```python
from build123d import *

# Parameters (mm, degrees)
SKETCH_1_R               = 32
SKETCH_1_R_2             = 2.5
SKETCH_1_R_3             = 1.25
EXTRUDE_1_DEPTH          = 20
SKETCH_2_R               = 2.75
CUT_EXTRUDE_1_DEPTH      = 2.1
SKETCH_3_R               = 2.5
CUT_EXTRUDE_2_DEPTH      = 3
SKETCH_4_R               = 1.65
CUT_EXTRUDE_3_DEPTH      = 10
PATTERN_CIRCULAR_1_COUNT = 6
SKETCH_5_R               = 15
CUT_EXTRUDE_4_DEPTH      = 21.0000001
SKETCH_6_R               = 2.75
SKETCH_6_R_2             = 1.25
CUT_EXTRUDE_5_DEPTH      = 3


with BuildPart() as part:
    # 草图1 → 凸台-拉伸1 (new body)
    with BuildSketch(Plane(origin=(0, 0, 0), x_dir=(1, 0, 0), z_dir=(0, 1, 0))):
        Circle(SKETCH_1_R)
        with Locations((-23.599192253, -13.625)):
            Circle(SKETCH_1_R_2, mode=Mode.SUBTRACT)
        with Locations((-13.625, -23.599192253)):
            Circle(SKETCH_1_R_3, mode=Mode.SUBTRACT)
        with Locations((0, -27.25)):
            Circle(SKETCH_1_R_2, mode=Mode.SUBTRACT)
        with Locations((13.625, -23.599192253)):
            Circle(SKETCH_1_R_3, mode=Mode.SUBTRACT)
        with Locations((23.599192253, -13.625)):
            Circle(SKETCH_1_R_2, mode=Mode.SUBTRACT)
        with Locations((27.25, 0)):
            Circle(SKETCH_1_R_3, mode=Mode.SUBTRACT)
        with Locations((23.599192253, 13.625)):
            Circle(SKETCH_1_R_2, mode=Mode.SUBTRACT)
        with Locations((13.625, 23.599192253)):
            Circle(SKETCH_1_R_3, mode=Mode.SUBTRACT)
        with Locations((0, 27.25)):
            Circle(SKETCH_1_R_2, mode=Mode.SUBTRACT)
        with Locations((-13.625, 23.599192253)):
            Circle(SKETCH_1_R_3, mode=Mode.SUBTRACT)
        with Locations((-23.599192253, 13.625)):
            Circle(SKETCH_1_R_2, mode=Mode.SUBTRACT)
        with Locations((-27.25, 0)):
            Circle(SKETCH_1_R_3, mode=Mode.SUBTRACT)
        with Locations((-23.599192253, -13.625)):
            Circle(SKETCH_1_R_2)
        with Locations((-23.599192253, 13.625)):
            Circle(SKETCH_1_R_2)
        with Locations((23.599192253, 13.625)):
            Circle(SKETCH_1_R_2)
        with Locations((0, 27.25)):
            Circle(SKETCH_1_R_2)
        with Locations((0, -27.25)):
            Circle(SKETCH_1_R_2)
        with Locations((23.599192253, -13.625)):
            Circle(SKETCH_1_R_2)
    extrude(amount=EXTRUDE_1_DEPTH)

    # 草图2 → 切除-拉伸1 (cut)
    with BuildSketch(Plane(origin=(0, 20, 0), x_dir=(1, 0, 0), z_dir=(0, 1, 0))):
        with Locations((-27.25, 0)):
            Circle(SKETCH_2_R)
        with Locations((13.625, 23.599192253)):
            Circle(SKETCH_2_R)
        with Locations((13.625, -23.599192253)):
            Circle(SKETCH_2_R)
    extrude(amount=-CUT_EXTRUDE_1_DEPTH, mode=Mode.SUBTRACT)

    # 草图3 → 切除-拉伸2 (cut)
    with BuildSketch(Plane(origin=(0, 20, 0), x_dir=(1, 0, 0), z_dir=(0, 1, 0))):
        with Locations((-19.55, 0)):
            Circle(SKETCH_3_R)
        with Locations((9.775, 16.930796644)):
            Circle(SKETCH_3_R)
        with Locations((9.775, -16.930796644)):
            Circle(SKETCH_3_R)
    extrude(amount=-CUT_EXTRUDE_2_DEPTH, mode=Mode.SUBTRACT)

    # 草图4 → 切除-拉伸3 (cut)
    with BuildSketch(Plane.XY.offset(32)):
        with Locations((0, 5)):
            Circle(SKETCH_4_R)
    cut_extrude_3 = extrude(amount=-CUT_EXTRUDE_3_DEPTH, mode=Mode.SUBTRACT)

    # 阵列(圆周)1: 切除-拉伸3 ×6 about axis
    pattern_circular_1_axis = Axis((0, 0, 0), (0, 1, 0))
    for i in range(1, PATTERN_CIRCULAR_1_COUNT):
        add(cut_extrude_3.rotate(pattern_circular_1_axis, i * 360 / PATTERN_CIRCULAR_1_COUNT), mode=Mode.SUBTRACT)

    # 草图5 → 切除-拉伸4 (cut, through all)
    with BuildSketch(Plane(origin=(0, 20, 0), x_dir=(1, 0, 0), z_dir=(0, 1, 0))):
        Circle(SKETCH_5_R)
    extrude(amount=-CUT_EXTRUDE_4_DEPTH, mode=Mode.SUBTRACT)

    # 草图6 → 切除-拉伸5 (cut)
    with BuildSketch(Plane.XZ):
        with Locations((13.625, -23.599192253)):
            Circle(SKETCH_6_R)
        with Locations((13.625, -23.599192253)):
            Circle(SKETCH_6_R_2, mode=Mode.SUBTRACT)
        with Locations((27.25, 0)):
            Circle(SKETCH_6_R)
        with Locations((27.25, 0)):
            Circle(SKETCH_6_R_2, mode=Mode.SUBTRACT)
        with Locations((13.625, 23.599192253)):
            Circle(SKETCH_6_R)
        with Locations((13.625, 23.599192253)):
            Circle(SKETCH_6_R_2, mode=Mode.SUBTRACT)
        with Locations((-13.625, 23.599192253)):
            Circle(SKETCH_6_R)
        with Locations((-13.625, 23.599192253)):
            Circle(SKETCH_6_R_2, mode=Mode.SUBTRACT)
        with Locations((-27.25, 0)):
            Circle(SKETCH_6_R)
        with Locations((-27.25, 0)):
            Circle(SKETCH_6_R_2, mode=Mode.SUBTRACT)
        with Locations((-13.625, -23.599192253)):
            Circle(SKETCH_6_R)
        with Locations((-13.625, -23.599192253)):
            Circle(SKETCH_6_R_2, mode=Mode.SUBTRACT)
    extrude(amount=-CUT_EXTRUDE_5_DEPTH, mode=Mode.SUBTRACT)


solid = part.part
```
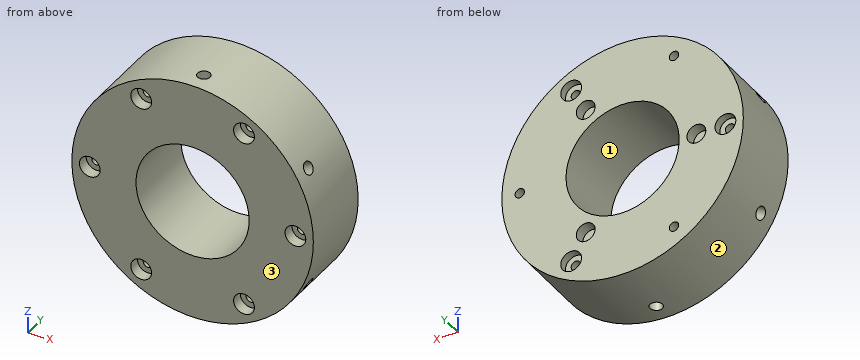
Input: part model. Units: mm. Frame: model coordinates. Face numbers are marked on the shaded views. Give positions to 0.01 mm unless a question says otherwise; leave off trailing zeros. Order: outer loops, then holes, each group sorted by start corner. A loop starts at its lowest first (then second) coordinate and runs counter-clockwise, first axis right, second up. Notation, with made-up numbers: M 64,36 L 123,36 A24 cw 123,49 Z; hole C -4.5,51 d6. An arc over 180 degrees is marked long. Return JSON: item names as keys, results as strings.
Item 1: Cut plane B-B (x = -0.5). Return loops of the section in (y, z), then the cut area to 3 significant figures.
Solutions:
{"outline": "M 0,-32 L 3.43,-32 L 3.43,-22 L 6.57,-22 L 6.57,-32 L 20,-32 L 20,-14.99 L 0,-14.99 Z; M 0,14.99 L 20,14.99 L 20,32 L 6.57,32 L 6.57,22 L 3.43,22 L 3.43,32 L 0,32 Z", "area": "617 mm^2"}
Item 2: First-contact query: P1, Ø4, axis at x = -4, y = 12.5, coming from the +Z side; P2, Ø3, axis at x = 13.62, z = 23.6, coming from the -Y side; P3, Ø10, axis at y = 2.5, z = 17.5, coming from the +X side. Flat tips, straight axial feed; report the tip coordinate or a pass-through.
Solutions:
{"P1": "z = 31.94", "P2": "y = 3", "P3": "x = 29.46"}
Item 3: Pull-direction query (Z, two-part tool) for the marked faces 1, 2 and 3; classes: +Z half, -Z half, draft (parallel to the pull), parting line (faces both ways), or undercut.
Solutions:
{"face 1": "undercut", "face 2": "parting line", "face 3": "draft"}
Item 4: Cut plane A-A (z = 0). State how many separate pieces and enclosed holes the cut face has, then the cut area to 3 significant figures.
Solutions:
{"separate pieces": "4", "enclosed holes": "0", "area": "541 mm^2"}
Item 5: Cut plane C-C (z = 8.5). Return loops of the section in (x, y), then the cut area to 3 significant figures.
Solutions:
{"outline": "M -30.85,0 L -12.36,0 L -12.36,20 L -30.85,20 Z; M 12.36,0 L 30.85,0 L 30.85,20 L 12.36,20 Z", "area": "740 mm^2"}
Item 6: Ray query, probe 1 along Z at (x, y) = (-13, 8.75); probe 2 along X at (y, z) = (2.25, 23.5); probe 3 along Z at (x, y) = (19.5, 5.25) (3 decimals). Return the intervals inside material, ascending.
Solutions:
{"probe 1": "-29.24 to -24.68, -22.52 to -7.48, 7.48 to 22.52, 24.68 to 29.24", "probe 2": "-21.72 to -16.37, -10.88 to 10.88, 16.37 to 21.72", "probe 3": "-25.372 to -13.142, -10.225 to 10.225, 13.142 to 25.372"}
Item 7: Cut plane D-D (y = 9). Return loops of the section in (x, z) (3 decimals).
Solutions:
{"outline": "C 0,0 d64; hole C -27.25,0 d2.5; hole C 0,0 d30; hole C -13.625,-23.599 d2.5; hole C -13.625,23.599 d2.5; hole C 13.625,-23.599 d2.5; hole C 13.625,23.599 d2.5; hole C 27.25,0 d2.5"}
